```python
from build123d import *

# Parameters (mm, degrees)
F0_R      = 23.5
F1_DEPTH  = 15
F3_DEPTH  = 25
F4_SIZE2  = 5
F4_SIZE   = 10
F5_SIZE2  = 5
F5_SIZE   = 10
F7_R      = 0.75
F8_DEPTH  = 12.5
F11_DEPTH = 5
F12_SIZE  = 0.5


with BuildPart() as f1:
    # F0 (on Top) → F1 (new body)
    with BuildSketch(Plane.XY):
        Circle(F0_R)
    extrude(amount=F1_DEPTH)

    # F2 (on face) → F3 (cut)
    with BuildSketch(Plane(origin=(0, 0, 0), x_dir=(1, 0, 0), z_dir=(0, 0, -1))):
        with BuildLine():
            ThreePointArc((0, -23.5), (-2.007337, -23.414111), (-4, -23.157072))
            Line((-4, -23.157072), (-4, -23.5))
            Line((-4, -23.5), (0, -23.5))
        make_face()
        with BuildLine():
            Line((4, -23.5), (4, -23.157072))
            ThreePointArc((4, -23.157072), (2.007337, -23.414111), (0, -23.5))
            Line((0, -23.5), (4, -23.5))
        make_face()
        with BuildLine():
            Line((-4, -15.5), (-4, -23.157072))
            ThreePointArc((-4, -23.157072), (-2.007337, -23.414111), (0, -23.5))
            Line((0, -23.5), (0, -15.5))
            Line((0, -15.5), (-4, -15.5))
        make_face()
        with BuildLine():
            ThreePointArc((0, -23.5), (2.007337, -23.414111), (4, -23.157072))
            Line((4, -23.157072), (4, -15.5))
            Line((4, -15.5), (0, -15.5))
            Line((0, -15.5), (0, -23.5))
        make_face()
        with BuildLine():
            ThreePointArc((4, 23.157072), (2.007337, 23.414111), (0, 23.5))
            Line((0, 23.5), (0, 15.5))
            Line((0, 15.5), (4, 15.5))
            Line((4, 15.5), (4, 23.157072))
        make_face()
        with BuildLine():
            Line((0, 15.5), (0, 23.5))
            ThreePointArc((0, 23.5), (-2.007337, 23.414111), (-4, 23.157072))
            Line((-4, 23.157072), (-4, 15.5))
            Line((-4, 15.5), (0, 15.5))
        make_face()
        with BuildLine():
            Line((4, 23.5), (0, 23.5))
            ThreePointArc((0, 23.5), (2.007337, 23.414111), (4, 23.157072))
            Line((4, 23.157072), (4, 23.5))
        make_face()
        with BuildLine():
            ThreePointArc((-4, 23.157072), (-2.007337, 23.414111), (0, 23.5))
            Line((0, 23.5), (-4, 23.5))
            Line((-4, 23.5), (-4, 23.157072))
        make_face()
    extrude(amount=-F3_DEPTH, mode=Mode.SUBTRACT)

    # F4
    f4_edges = [f1.edges().sort_by_distance(p)[0] for p in [
        (0, -15.5, 15),
    ]]
    chamfer(f4_edges, length=F4_SIZE, length2=F4_SIZE2)

    # F5
    f5_edges = [f1.edges().sort_by_distance(p)[0] for p in [
        (0, 15.5, 15),
    ]]
    chamfer(f5_edges, length=F5_SIZE, length2=F5_SIZE2)

    # F7 (on Right) → F8 (cut, symmetric)
    with BuildSketch(Plane.YZ):
        with Locations((-21.157072, 3)):
            Circle(F7_R)
        with Locations((21.157072, 3)):
            Circle(F7_R)
    extrude(amount=F8_DEPTH, both=True, mode=Mode.SUBTRACT)

    # F10 (on face) → F11 (cut)
    with BuildSketch(Plane.XY.offset(15)):
        with BuildLine():
            ThreePointArc((-12.5, 10.763446), (-11.272071, 11.272071), (-10.763446, 12.5))
            Line((-10.763446, 12.5), (-12.5, 12.5))
            Line((-12.5, 12.5), (-12.5, 10.763446))
        make_face()
        with BuildLine():
            Line((-12.5, 12.5), (-10.763446, 12.5))
            ThreePointArc((-10.763446, 12.5), (-13.727929, 13.727929), (-12.5, 10.763446))
            Line((-12.5, 10.763446), (-12.5, 12.5))
        make_face()
        with BuildLine():
            ThreePointArc((-10.763446, -12.5), (-11.272071, -11.272071), (-12.5, -10.763446))
            Line((-12.5, -10.763446), (-12.5, -12.5))
            Line((-12.5, -12.5), (-10.763446, -12.5))
        make_face()
        with BuildLine():
            Line((-12.5, -12.5), (-12.5, -10.763446))
            ThreePointArc((-12.5, -10.763446), (-13.727929, -13.727929), (-10.763446, -12.5))
            Line((-10.763446, -12.5), (-12.5, -12.5))
        make_face()
        with BuildLine():
            Line((12.5, -12.5), (12.5, -10.763446))
            ThreePointArc((12.5, -10.763446), (11.272071, -11.272071), (10.763446, -12.5))
            Line((10.763446, -12.5), (12.5, -12.5))
        make_face()
        with BuildLine():
            Line((12.5, 12.5), (10.763446, 12.5))
            ThreePointArc((10.763446, 12.5), (11.272071, 11.272071), (12.5, 10.763446))
            Line((12.5, 10.763446), (12.5, 12.5))
        make_face()
        with BuildLine():
            ThreePointArc((14.236554, 12.5), (12.5, 14.236554), (10.763446, 12.5))
            Line((10.763446, 12.5), (12.5, 12.5))
            Line((12.5, 12.5), (12.5, 10.763446))
            ThreePointArc((12.5, 10.763446), (13.727929, 11.272071), (14.236554, 12.5))
        make_face()
        with BuildLine():
            ThreePointArc((14.236554, -12.5), (13.727929, -11.272071), (12.5, -10.763446))
            Line((12.5, -10.763446), (12.5, -12.5))
            Line((12.5, -12.5), (10.763446, -12.5))
            ThreePointArc((10.763446, -12.5), (12.5, -14.236554), (14.236554, -12.5))
        make_face()
    extrude(amount=-F11_DEPTH, mode=Mode.SUBTRACT)

    # F12
    f12_edges = [f1.edges().sort_by_distance(p)[0] for p in [
        (23.5, 0, 0),
        (4, 19.328536, 0),
        (0, 15.5, 0),
        (-4, 19.328536, 0),
        (-23.5, 0, 0),
        (-4, -19.328536, 0),
        (0, -15.5, 0),
        (4, -19.328536, 0),
    ]]
    chamfer(f12_edges, length=F12_SIZE)


solid = f1.part
```
For this review, take the finished solid that the model builds, in its own axes (mm). A direction names the side the tool comes from. Coordinates: 2 decimals unless noted, no trailing zeros. Loops run counter-clockwise (first coordinate to the right, second up) from the corner with the lowest first, then second, coordinate; pieces in that order, holes last. Notation, with made-up numbers: (37, 2.5) -> (50, 2.5) arc R13 ccw to (50, 17.5) -> close; hole circle Ø7 at (-18.5, 74). An arc over 180 degrees is marked (long way). Return JSON: item names as keys, results as strings. Group by question number.
(1) Consider section C-C, the plane z = 6.75. Give the boundary of the cut face in (x, y) (3 decimals).
(2) Consider section A-A, the plane z = 12.5. Give the boundary of the cut face in (x, y).
(3) For pin 1 Ø5 at (x, z) = (1, 2) entering from +Y; pin 2 Ø6.5 at (y, z) = (-17.5, 4) entering from -X; pin 3 Ø1.3 at (x, z) = (-1.5, 2) entering from -Y, all flat-tipped, find the tip position at first contact; note any pin that passes through.
(4) To check wall thickness, follow L1, parallel to Y at x = -5.5, z = 3; L2, parallel to Y at x = -12.5, z = 12.1; L3, parallel to X at y = 12.5, z = 13. State the ranges of each line that lie inside material, in increasing order.
(5) Mouldability with a two-part tool opening along Z and no side actions: class faces 1 (the cylindrical face through (-6.923, 20.408, 3.033)), 2 (the flat face through (4, 18, 8)), 3 (the flat face through (-13, 13, 10)) as pulls with the +Z half, pulls with the -Z half, needs draft (parallel to the pull), parting line crosses it, or undercut.
(6) Tool access review of faces 4 (the flat face through (0, 15.5, 3)), 5 (the flat face through (0, -13, 10)), 6 (the flat face through (12, 13, 10)), 7 (the flat face through (0, 13, 10)): name each direction out of +Z, -Z, +X, -X, +Y, -Y from which nothing blocks a thin tool from reaching the whole face with its end or side.
(7) Consider section B-B, the plane z = 1.5. Give the boundary of the cut face in (x, y), plus the area to 3 significant figures.
Results below:
{
 "1": {"outline": "(-4, -23.157) -> (-4, -14.625) -> (4, -14.625) -> (4, -23.157) arc R23.5 ccw to (4, 23.157) -> (4, 14.625) -> (-4, 14.625) -> (-4, 23.157) arc R23.5 ccw to start"},
 "2": {"outline": "(-4, -23.16) -> (-4, -11.75) -> (4, -11.75) -> (4, -23.16) arc R23.5 ccw to (4, 23.16) -> (4, 11.75) -> (-4, 11.75) -> (-4, 23.16) arc R23.5 ccw to start; hole circle Ø3.47 at (-12.5, -12.5); hole circle Ø3.47 at (-12.5, 12.5); hole circle Ø3.47 at (12.5, -12.5); hole circle Ø3.47 at (12.5, 12.5)"},
 "3": {"pin 1": "stops at y = 15.5", "pin 2": "stops at x = -18.69", "pin 3": "stops at y = -15.5"},
 "4": {"L1": "y = -22.85 to -21.91, -20.41 to 20.41, 21.91 to 22.85", "L2": "y = -19.9 to -14.24, -10.76 to 10.76, 14.24 to 19.9", "L3": "x = -19.9 to -14.24, -10.76 to -4, 4 to 10.76, 14.24 to 19.9"},
 "5": {"face 1": "undercut", "face 2": "needs draft", "face 3": "pulls with the +Z half"},
 "6": {"face 4": "+Z, -Z, +Y", "face 5": "+Z, -Y", "face 6": "+Z", "face 7": "+Z, +Y"},
 "7": {"outline": "(-4, -23.16) -> (-4, -15.5) -> (4, -15.5) -> (4, -23.16) arc R23.5 ccw to (4, 23.16) -> (4, 15.5) -> (-4, 15.5) -> (-4, 23.16) arc R23.5 ccw to start", "area": "1,610 mm2"}
}
